Verification items for the finished model (mm, model axes). Round coordinates to 2 decimals unless told otherwise and drop trailing zeros. Loops run counter-clockwise (first coordinate to the right, second up) from the corner with the lowest first, then second, coordinate; pieces in that order, holes last. Notation, with made-up numbers: (-2.75, -23.75) -> (18.25, -23.75) arc R14 ccw to (18.25, -0.75) -> close; hole circle Ø8 at (-24, 23.25). An arc over 180 degrees is marked (long way). Write item = value, one per line.
Solid Edge part; units mm, degrees
sketch "Sketch1" plane through (0, 0, 0) normal (0, 0, 1) x (1, 0, 0)
  line L0 (-16, -30) -> (16, -30)
  line L1 (16, -30) -> (16, 30)
  line L2 (16, 30) -> (-16, 30)
  line L3 (-16, 30) -> (-16, -30)
  dimension "D1" = 16
  dimension "D2" = 16
extrude "Protrusion1" add sketch "Sketch1" along normal blind 73
sketch "Sketch2" plane through (0, 0, 73) normal (0, 0, 1) x (1, 0, 0)
  circle A0 centre (0, -20) radius 2.35
  circle A1 centre (0, -2) radius 2.35
extrude "Cutout1" cut sketch "Sketch2" against normal through all
chamfer "Fase_3" distance 0.7 angle 60 4 edges at (-2.35, -2, 73) (-2.35, -20, 73) (-2.35, -20, 0) (-2.35, -2, 0) measured on face at (-10.9867, -19.4, 73) measured on face at (-10.9867, -19.4, 0)
chamfer "Fase_6" distance 3 angle 45 4 edges at (-16, 0, 73) (-16, 0, 0) (16, 0, 73) (16, 0, 0)
chamfer "Fase_7" distance 3 angle 45 2 edges at (0, -30, 73) (0, -30, 0)
sketch "Sketch3" plane through (-16, 0, 36.5) normal (-1, 0, 0) x (0, -1, 0)
  circle A0 centre (-20, 25) radius 2.35
  circle A1 centre (-20, -25) radius 2.35
  circle A2 centre (10, 0) radius 2.35
  dimension "D1" = 20
extrude "Cutout2" cut sketch "Sketch3" against normal through all
chamfer "Fase_9" distance 0.7 angle 60 6 edges at (-16, 22.35, 61.5) (-16, -7.65, 36.5) (-16, 22.35, 11.5) (16, 20, 59.15) (16, 20, 9.15) (16, -10, 34.15) measured on face at (-16, 20.6, 58.1633) measured on face at (16, -20.6, 58.1633)
sketch "Sketch4" plane through (-16, 0, 36.5) normal (-1, 0, 0) x (0, -1, 0)
  line L0 (-6.5, 36.5) -> (-30, 36.5)
  line L1 (-30, 36.5) -> (-30, 36)
  line L2 (-30, 36) -> (-6.5, 36)
  line L3 (-6.5, 36) -> (-6.5, 36.5)
  line L4 (-30, -36.5) -> (-6.5, -36.5)
  line L5 (-6.5, -36.5) -> (-6.5, -36)
  line L6 (-6.5, -36) -> (-30, -36)
  line L7 (-30, -36) -> (-30, -36.5)
  dimension "D1" = 30
  dimension "D2" = 30
extrude "Cutout3" cut sketch "Sketch4" against normal through all
sketch "Sketch5" plane through (0, 30, 36.5) normal (0, 1, 0) x (1, 0, 0)
  line L0 (-16, 33.5) -> (-13.5, 36)
  line L1 (-13.5, 36) -> (13.5, 36)
  line L2 (13.5, 36) -> (16, 33.5)
  line L3 (16, 33.5) -> (16, -33.5)
  line L4 (16, -33.5) -> (13.5, -36)
  line L5 (13.5, -36) -> (-13.5, -36)
  line L6 (-13.5, -36) -> (-16, -33.5)
  line L7 (-16, -33.5) -> (-16, 33.5)
extrude "Protrusion2" add sketch "Sketch5" along normal blind 26
sketch "Sketch6" plane through (0, 36.25, 72.5) normal (0, 0, 1) x (0, 1, 0)
  circle A0 centre (11.75, 0) radius 2.35
  dimension "D1" = 11.75
extrude "Cutout4" cut sketch "Sketch6" against normal through all
chamfer "Fase_10" distance 0.7 angle 60 2 edges at (0, 45.65, 72.5) (-2.35, 48, 0.5) measured on face at (8.73, 48.245, 72.5) measured on face at (8.73, 14.255, 0.5)
sketch "Sketch7" plane through (0, 56, 36.5) normal (0, 1, 0) x (-1, 0, 0)
  line L0 (-13.5, 36) -> (-16, 33.5)
  line L1 (-16, 33.5) -> (-16, -33.5)
  line L2 (-16, -33.5) -> (-13.5, -36)
  line L3 (-13.5, -36) -> (13.5, -36)
  line L4 (13.5, -36) -> (16, -33.5)
  line L5 (16, -33.5) -> (16, 33.5)
  line L6 (16, 33.5) -> (13.5, 36)
  line L7 (13.5, 36) -> (-13.5, 36)
extrude "Extrusionsausprägung_3" add sketch "Sketch7" along normal blind 6
properties material "Nylon, allgemein"
(1) Material ranges on probe 1 along Y at (x, z) = (0, 34); probe 2 along Z at (x, y) = (-3, 20); probe 3 along Z at (x, y) = (3, -10), recorded low to high. Write a range as from..to.
Filled sheet:
probe_1 = -30..-22.35, -17.65..-4.35, 0.35..45.65, 50.35..62
probe_2 = 0.5..9.15, 13.85..59.15, 63.85..72.5
probe_3 = 0..34.15, 38.85..73
(2) Sectioned sample at D-D, the plane x = -9.5. Record the cut outline in (y, z), and give its area (3 significant figures).
Filled sheet:
outline = (-30, 3) -> (-27, 0) -> (6.5, 0) -> (6.5, 0.5) -> (62, 0.5) -> (62, 72.5) -> (6.5, 72.5) -> (6.5, 73) -> (-27, 73) -> (-30, 70) -> close; hole circle Ø4.7 at (-10, 36.5); hole circle Ø4.7 at (20, 11.5); hole circle Ø4.7 at (20, 61.5)
area = 6,600 mm2
(3) Sectioned sample at C-C, the plane y = 20. Record the cut outline in (x, z), and give its area (3 significant figures).
Filled sheet:
outline = (-16, 3) -> (-13.5, 0.5) -> (13.5, 0.5) -> (16, 3) -> (16, 8.45) -> (14.79, 9.15) -> (-14.79, 9.15) -> (-16, 8.45) -> close; (-16, 14.55) -> (-14.79, 13.85) -> (14.79, 13.85) -> (16, 14.55) -> (16, 58.45) -> (14.79, 59.15) -> (-14.79, 59.15) -> (-16, 58.45) -> close; (-16, 64.55) -> (-14.79, 63.85) -> (14.79, 63.85) -> (16, 64.55) -> (16, 70) -> (13.5, 72.5) -> (-13.5, 72.5) -> (-16, 70) -> close
area = 1,990 mm2
(4) Draft check along X on faces 1 (the face through (16, 15, 36)), 2 (the face through (0, 34, 72.5)), 3 (the face through (-0.509, -22.294, 36.994)), 4 (the face through (-16, 17, 36)). Enter one of: released by +X, released by -X, zero draft, split by the parting line, or undercut.
Filled sheet:
face_1 = released by +X
face_2 = zero draft
face_3 = undercut
face_4 = released by -X
(5) Sectioned sample at B-B, the plane z = 36.5. Record the cut outline in (x, y).
Filled sheet:
outline = (-16, -30) -> (16, -30) -> (16, -13.05) -> (14.79, -12.35) -> (-14.79, -12.35) -> (-16, -13.05) -> close; (-16, -6.95) -> (-14.79, -7.65) -> (14.79, -7.65) -> (16, -6.95) -> (16, 62) -> (-16, 62) -> close; hole circle Ø4.7 at (0, -20); hole circle Ø4.7 at (0, -2); hole circle Ø4.7 at (0, 48)
(6) Sectioned sample at A-A, the plane y = -20. Record the cut outline in (x, z), and give its area (3 significant figures).
Filled sheet:
outline = (-16, 3) -> (-13, 0) -> (-3.05, 0) -> (-2.35, 1.21) -> (-2.35, 71.79) -> (-3.05, 73) -> (-13, 73) -> (-16, 70) -> close; (2.35, 1.21) -> (3.05, 0) -> (13, 0) -> (16, 3) -> (16, 70) -> (13, 73) -> (3.05, 73) -> (2.35, 71.79) -> close
area = 1,970 mm2
(7) Go/stop test with flat-tipped pins: pin 1 Ø5.5 at (x, y) = (0, -2) entering from -Z; pin 2 Ø3 at (y, z) = (20, 11.5) entering from -X; pin 3 Ø8 at (x, y) = (5, 32.5) entering from +Z; pin 4 Ø0.6 at (x, z) = (-3.5, 0) entering from +Y. Record where each tip stops, or that it passes through.
Filled sheet:
pin_1 = 0.52
pin_2 = through
pin_3 = 72.5
pin_4 = 6.5
